```python
from build123d import *

# Parameters (mm, degrees)
SKETCH1_W           = 34
SKETCH1_H           = 58
BOSS_EXTRUDE1_DEPTH = 13
SKETCH3_W           = 4.5
SKETCH3_H           = 13
CUT_EXTRUDE1_DEPTH  = 2.7
SKETCH5_R           = 4.3
CUT_EXTRUDE2_DEPTH  = 36.158071619
SKETCH12_W          = 4.5
SKETCH12_H          = 13
CUT_EXTRUDE3_DEPTH  = 45
CUT_EXTRUDE4_DEPTH  = 37.041642582
SKETCH9_R           = 1.05
CUT_EXTRUDE6_DEPTH  = 13
CUT_EXTRUDE7_DEPTH  = 5.5
SKETCH13_W          = 34
SKETCH13_H          = 5
CUT_EXTRUDE8_DEPTH  = 15


with BuildPart() as part:
    # Sketch1 → Boss-Extrude1 (new body)
    with BuildSketch(Plane(origin=(0, 0, 0), x_dir=(1, 0, 0), z_dir=(0, 1, 0))):
        Rectangle(SKETCH1_W, SKETCH1_H)
    extrude(amount=BOSS_EXTRUDE1_DEPTH)

    # Sketch3 → Cut-Revolve1 (revolve, cut)
    with BuildSketch(Plane(origin=(0, 0, 0), x_dir=(0, 0, -1), z_dir=(1, 0, 0)), mode=Mode.PRIVATE) as cut_revolve1_sk:
        with Locations((-14.75, 6.5)):
            Rectangle(SKETCH3_W, SKETCH3_H)
    revolve(cut_revolve1_sk.sketch.rotate(Axis((0, 13, 17), (0, -1, 0)), 180), axis=Axis((0, 13, 17), (0, -1, 0)), mode=Mode.SUBTRACT)

    # Sketch4 → Cut-Extrude1 (cut)
    with BuildSketch(Plane.XZ):
        Polygon((3.70947548, -5.425), (7.418950959, 1), (3.70947548, 7.425), (-3.70947548, 7.425), (-7.418950959, 1), (-3.70947548, -5.425), align=None)
    extrude(amount=-CUT_EXTRUDE1_DEPTH, mode=Mode.SUBTRACT)

    # Sketch5 → Cut-Extrude2 (cut, through all)
    with BuildSketch(Plane.XZ.offset(-2.7)):
        with Locations(Location((0, 1, 0), (0, 0, 270))):
            Circle(SKETCH5_R)
    extrude(amount=-CUT_EXTRUDE2_DEPTH, mode=Mode.SUBTRACT)

    # Sketch12 → Cut-Revolve2 (revolve, cut)
    with BuildSketch(Plane(origin=(0, 0, 0), x_dir=(0, 0, -1), z_dir=(1, 0, 0))):
        with Locations((17.25, 6.5)):
            Rectangle(SKETCH12_W, SKETCH12_H)
    revolve(axis=Axis((0, 0, -15), (0, 1, 0)), mode=Mode.SUBTRACT)

    # Sketch6 → Cut-Extrude3 (cut)
    with BuildSketch(Plane(origin=(0, 0, -29), x_dir=(-1, 0, 0), z_dir=(0, 0, -1))):
        Polygon((-17, 6), (-14, 6), (-14, 9), (-6.699377385, 9), (-8.8, 6), (-8.8, 0), (-17, 0), align=None)
        Polygon((8.8, 0), (17, 0), (17, 6), (14, 6), (14, 9), (6.699377385, 9), (8.8, 6), align=None)
    extrude(amount=-CUT_EXTRUDE3_DEPTH, mode=Mode.SUBTRACT)

    # Sketch7 → Cut-Extrude4 (cut, through all)
    with BuildSketch(Plane(origin=(0, 13, 0), x_dir=(1, 0, 0), z_dir=(0, 1, 0))):
        with BuildLine():
            Line((17, -29), (17, -18.253317763))
            ThreePointArc((17, -18.253317763), (10.05598304, -26.088042865), (1.4e-08, -29))
            Line((1.4e-08, -29), (17, -29))
        make_face()
        with BuildLine():
            Line((-17, -29), (1.4e-08, -29))
            ThreePointArc((1.4e-08, -29), (-10.055983028, -26.088042873), (-17, -18.253317763))
            Line((-17, -18.253317763), (-17, -29))
        make_face()
    extrude(amount=-CUT_EXTRUDE4_DEPTH, mode=Mode.SUBTRACT)

    # Sketch9 → Cut-Extrude6 (cut)
    with BuildSketch(Plane.XZ):
        with Locations(Location((0, -7, 0), (0, 0, 270))):
            Circle(SKETCH9_R)
        with Locations(Location((0, 9, 0), (0, 0, 270))):
            Circle(SKETCH9_R)
    extrude(amount=-CUT_EXTRUDE6_DEPTH, mode=Mode.SUBTRACT)

    # Sketch10 → Cut-Extrude7 (cut)
    with BuildSketch(Plane(origin=(0, 13, 0), x_dir=(1, 0, 0), z_dir=(0, 1, 0))):
        Polygon((0, -6.546261356), (-2.125, -7.773130678), (-2.125, -10.226869322), (0, -11.453738644), (2.125, -10.226869322), (2.125, -7.773130678), align=None)
        Polygon((0, 9.453738644), (-2.125, 8.226869322), (-2.125, 5.773130678), (0, 4.546261356), (2.125, 5.773130678), (2.125, 8.226869322), align=None)
    extrude(amount=-CUT_EXTRUDE7_DEPTH, mode=Mode.SUBTRACT)

    # Sketch13 → Cut-Extrude8 (cut)
    with BuildSketch(Plane(origin=(0, 13, 0), x_dir=(1, 0, 0), z_dir=(0, 1, 0))):
        with Locations((0, 26.5)):
            Rectangle(SKETCH13_W, SKETCH13_H)
    extrude(amount=-CUT_EXTRUDE8_DEPTH, mode=Mode.SUBTRACT)


solid = part.part
```
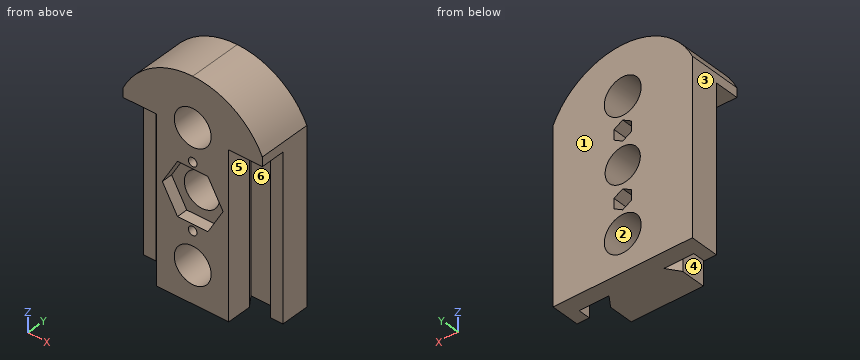
For this review, take the finished solid that the model builds, in its own axes (mm). Face numbers are marked on the shaded views. A direction names the side the tool comes from. Coordinates: 2 decimals unless noted, no trailing zeros. Write each loop counter-clockwise with the first axis right and the second up, starting at its lowest first coordinate (ties: lowest second). Pieces come first, ordered by that corner, then holes.
(1) Add section B-B on y = 12. Give the boundary of the cut face in (x, z) (3 decimals).
(2) Wall thickness on probe 1 along X at (y, z) = (3, 9); probe 2 along X at (y, z) = (7, 1); probe 3 along X at (y, z) = (4.5, 17): over which ranges is each line inside the solid? List them lowest first.
(3) Tool access review of the marked faces 4, 5 and 6: name each direction out of +Z, -Z, +X, -X, +Y, -Y from which nothing blocks a thin tool from reaching the whole face with its end or side.
(4) For pin 1 Ø14 at (x, z) = (0, 1) entering from -Y; pin 2 Ø5 at (y, z) = (2, -9) entering from -X; pin 3 Ø2 at (y, z) = (4, 5.5) entering from +X; pin 4 Ø0.9 at (x, z) = (-16, 1.5) entering from -Y, all flat-tipped, find the tip position at first contact; note any pin that passes through.
(5) Add section A-A on z = 9. Give the boundary of the cut face in (x, y) (3 decimals), then the cut area to 3 significant figures.
(6) Add section C-C on z = 17. Give the boundary of the cut face in (x, y), then the cut area to 3 significant figures.
(7) The part is to be moulded in two halves that separate along X. For the marked faces 1, 2 and 3, say which applies: +X half, -X half, draft (parallel to the pull), parting line (faces both ways), or undercut.
(8) Add section D-D on y = 4. Give the boundary of the cut face in (x, z).
Answer sheet:
1. outline: (-17, -24) - (17, -24) - (17, 18.253) arc R18.819 ccw to (-17, 18.253) - close; hole circle Ø9 at (0, -15); hole circle Ø9 at (0, 17); hole circle Ø8.6 at (0, 1); hole (-2.125, -8.227) - (0, -9.454) - (2.125, -8.227) - (2.125, -5.773) - (0, -4.546) - (-2.125, -5.773) - close; hole (-2.125, 7.773) - (0, 6.546) - (2.125, 7.773) - (2.125, 10.227) - (0, 11.454) - (-2.125, 10.227) - close
2. probe 1: x = -8.8 to -1.05, 1.05 to 8.8
2. probe 2: x = -17 to -14, -8.1 to -4.3, 4.3 to 8.1, 14 to 17
2. probe 3: x = -17 to -4.5, 4.5 to 17
3. face 4: -Z, -X, -Y
3. face 5: -Z, +X, -Y
3. face 6: -Z
4. pin 1: stops at y = 0
4. pin 2: stops at x = -8.8
4. pin 3: stops at x = 8.8
4. pin 4: stops at y = 6
5. outline: (-17, 6) - (-14, 6) - (-14, 9) - (-6.699, 9) - (-8.8, 6) - (-8.8, 0) - (-1.05, 0) - (-1.05, 7.5) - (-2.125, 7.5) - (-2.125, 13) - (-17, 13) - close; (1.05, 0) - (8.8, 0) - (8.8, 6) - (6.699, 9) - (14, 9) - (14, 6) - (17, 6) - (17, 13) - (2.125, 13) - (2.125, 7.5) - (1.05, 7.5) - close
5. area: 267 mm2
6. outline: (-17, 0) - (-4.5, 0) - (-4.5, 13) - (-17, 13) - close; (4.5, 0) - (17, 0) - (17, 13) - (4.5, 13) - close
6. area: 325 mm2
7. face 1: draft
7. face 2: undercut
7. face 3: -X half
8. outline: (-17, 16) - (-8.8, 16) - (-8.8, -24) - (8.8, -24) - (8.8, 16) - (17, 16) - (17, 18.25) arc R18.82 ccw to (-17, 18.25) - close; hole circle Ø9 at (0, -15); hole circle Ø9 at (0, 17); hole circle Ø8.6 at (0, 1); hole circle Ø2.1 at (0, -7); hole circle Ø2.1 at (0, 9)
